Can you work these out from the model? Positions are in its coordinate system, mm. A direction names the side the tool comes from. Give positions to 0.01 mm unless a question says otherwise; leave off trailing zeros. Write each loop counter-clockwise with the first axis right and the second up, starting at its lowest first coordinate (ties: lowest second). Pieces come first, ordered by that corner, then holes. Notation, with made-up numbers: (-36, 81) - (-2, 81) arc R22 cw to (-2, 112) - close; hole circle Ø11 at (4, 17). An arc over 180 degrees is marked (long way). Use a Markdown table: item, result. Add a question column.
```python
from build123d import *

# Parameters (mm, degrees)
SKETCH2_R           = 20.1
BOSS_EXTRUDE2_DEPTH = 3
BOSS_EXTRUDE4_DEPTH = 10.9
FILLET1_R           = 2
FILLET2_R           = 1


with BuildPart() as part:
    # Sketch2 → Boss-Extrude2 (new body)
    with BuildSketch(Plane(origin=(0, 0, 0), x_dir=(1, 0, 0), z_dir=(0, 1, 0))):
        with Locations(Location((0, 0, 0), (0, 0, 270))):
            Circle(SKETCH2_R)
    extrude(amount=BOSS_EXTRUDE2_DEPTH)

    # Sketch3 → Boss-Extrude4 (add)
    with BuildSketch(Plane(origin=(0, 3, 0), x_dir=(1, 0, 0), z_dir=(0, 1, 0))):
        Polygon((-4.943443761, 18.449183282), (-4.555215194, 17.000294543), (-4.555215194, 14.000294543), (4.555215194, 14.000294543), (4.555215194, 17.000294543), (4.943443761, 18.449183282), (2.054487352, 18.989183282), (-2.054487352, 18.989183282), align=None)
        Polygon((17.000294543, 4.555215194), (14.000294543, 4.555215194), (14.000294543, -4.555215194), (17.000294543, -4.555215194), (18.449183282, -4.943443761), (18.989183282, -2.054487352), (18.989183282, 2.054487352), (18.449183282, 4.943443761), align=None)
        Polygon((-17.000294543, -4.555215194), (-14.000294543, -4.555215194), (-14.000294543, 4.555215194), (-17.000294543, 4.555215194), (-18.449183282, 4.943443761), (-18.989183282, 2.054487352), (-18.989183282, -2.054487352), (-18.449183282, -4.943443761), align=None)
    extrude(amount=BOSS_EXTRUDE4_DEPTH)

    # Fillet1
    fillet1_edges = [part.edges().sort_by_distance(p)[0] for p in [
        (-14.000294543, 3, 0),
        (14.000294543, 3, 0),
        (0, 3, -14.000294543),
    ]]
    fillet(fillet1_edges, radius=FILLET1_R)

    # Fillet2
    fillet2_edges = [part.edges().sort_by_distance(p)[0] for p in [
        (0, 0, -20.1),
    ]]
    fillet(fillet2_edges, radius=FILLET2_R)


solid = part.part
```
Q1. Suppose I cut it at B-B (z = 0). Please give me the cut outline in (x, y), and give its area (3 significant figures).
Q2. Suppose I cut it at A-A (y = 7). Please give me the cut outline in (x, z).
Q3. If I drill on probe 1 along Y at (x, z) = (6.5, -2); probe 2 along X at (y, z) = (6.5, -14.5), over which ranges is the centre line in solid material (lowest first)? Write a range as [from, to].
Q4. Suppose I cut it at C-C (x = 0). Please give me the cut outline in (y, z).
Q5. I'm going to push flat-ended pins straight in: P1, Ø5.5, axis at x = 14.5, y = 7, coming from the +Z side; P2, Ø3.5, axis at y = 8, z = 0, coming from the -X side; P3, Ø4.5, axis at y = 10.5, z = -1, coming from the +X side. Where does each tip first touch, or does it pass through?
Q6. On a 3-axis mill with a long thin cutter (end or side, diameter ignored), from which of +Z, -Z, +X, -X, +Y, -Y can I reach the whole of each face in a straight line? I mean faces 1 (the flat face through (-4.555, 8, -16)), 2 (the flat face through (4.555, 8, -16)), 3 (the flat face through (-16, 8, -4.555)). Say none if no direction works.
Q7. If we mould it in two halves opening along X, with no side actions, what happens to faces 4 (the flat face through (-14, 9, 0)), 5 (the flat face through (0, 9, -14)), 6 (the flat face through (3.519, 8.374, -18.715))? For each: released by +X, released by -X, zero draft, split by the parting line, or undercut.
Derived:
| question | item | result |
|---|---|---|
| 1 | outline | (-20.1, 1) arc R1 ccw to (-19.1, 0) - (19.1, 0) arc R1 ccw to (20.1, 1) - (20.1, 3) - (18.99, 3) - (18.99, 13.9) - (14, 13.9) - (14, 5) arc R2 cw to (12, 3) - (-12, 3) arc R2 cw to (-14, 5) - (-14, 13.9) - (-18.99, 13.9) - (-18.99, 3) - (-20.1, 3) - close |
| 1 | area | 231 mm² |
| 2 | outline | (-18.99, -2.05) - (-18.45, -4.94) - (-17, -4.56) - (-14, -4.56) - (-14, 4.56) - (-17, 4.56) - (-18.45, 4.94) - (-18.99, 2.05) - close; (-4.94, -18.45) - (-2.05, -18.99) - (2.05, -18.99) - (4.94, -18.45) - (4.56, -17) - (4.56, -14) - (-4.56, -14) - (-4.56, -17) - close; (14, -4.56) - (17, -4.56) - (18.45, -4.94) - (18.99, -2.05) - (18.99, 2.05) - (18.45, 4.94) - (17, 4.56) - (14, 4.56) - close |
| 3 | probe 1 | [0, 3] |
| 3 | probe 2 | [-4.56, 4.56] |
| 4 | outline | (0, -19.1) arc R1 ccw to (1, -20.1) - (3, -20.1) - (3, -18.99) - (13.9, -18.99) - (13.9, -14) - (5, -14) arc R2 cw to (3, -12) - (3, 20.1) - (1, 20.1) arc R1 ccw to (0, 19.1) - close |
| 5 | P1 | z = 4.62 |
| 5 | P2 | x = -18.99 |
| 5 | P3 | x = 18.99 |
| 6 | face 1 | +Z, -X, +Y |
| 6 | face 2 | +Z, +X, +Y |
| 6 | face 3 | -Z, +Y |
| 7 | face 4 | undercut |
| 7 | face 5 | zero draft |
| 7 | face 6 | released by +X |
